```python
from build123d import *

# Parameters (mm, degrees)
SKETCH1_R           = 8.255
SKETCH1_R_2         = 5.715
BOSS_EXTRUDE1_DEPTH = 269.875
CUT_EXTRUDE1_DEPTH  = 271.127387865
SKETCH3_R           = 1.524
CUT_EXTRUDE2_DEPTH  = 271.127387865
SKETCH4_R           = 5.715
SKETCH4_R_2         = 5.08
BOSS_EXTRUDE2_DEPTH = 3.81


with BuildPart() as part:
    # Sketch1 → Boss-Extrude1 (new body)
    with BuildSketch(Plane(origin=(0, 0, 0), x_dir=(1, 0, 0), z_dir=(0, 1, 0))):
        with Locations(Location((0, 0, 0), (0, 0, 270))):
            Circle(SKETCH1_R)
        with Locations(Location((0, 0, 0), (0, 0, 270))):
            Circle(SKETCH1_R_2, mode=Mode.SUBTRACT)
    extrude(amount=BOSS_EXTRUDE1_DEPTH)

    # Sketch2 → Cut-Extrude1 (cut, through all)
    with BuildSketch(Plane(origin=(0, 0, 0), x_dir=(0, 0, -1), z_dir=(1, 0, 0))):
        Polygon((1.833087105, 260.35), (3.666174209, 263.525), (1.833087105, 266.7), (-1.833087105, 266.7), (-3.666174209, 263.525), (-1.833087105, 260.35), align=None)
    extrude(amount=-CUT_EXTRUDE1_DEPTH, mode=Mode.SUBTRACT)

    # Sketch3 → Cut-Extrude2 (cut, through all)
    with BuildSketch(Plane(origin=(0, 0, 0), x_dir=(0, 0, -1), z_dir=(1, 0, 0))):
        with Locations(Location((0, 263.525, 0), (0, 0, 180))):
            Circle(SKETCH3_R)
    extrude(amount=CUT_EXTRUDE2_DEPTH, mode=Mode.SUBTRACT)

    # Sketch4 → Boss-Extrude2 (add)
    with BuildSketch(Plane.XZ):
        with Locations(Location((0, 0, 0), (0, 0, 270))):
            Circle(SKETCH4_R)
        with Locations(Location((0, 0, 0), (0, 0, 270))):
            Circle(SKETCH4_R_2, mode=Mode.SUBTRACT)
    extrude(amount=-BOSS_EXTRUDE2_DEPTH)


solid = part.part
```
Geometry: final body of the model. Coordinates: model frame, mm. A direction names the side the tool comes from. Give positions to 0.01 mm unless a question says otherwise; leave off trailing zeros. Order: outer loops, then holes, each group sorted by start corner. A loop starts at its lowest first (then second) coordinate and runs counter-clockwise, first axis right, second up. Notation, with made-up numbers: (-18.5, 80.5) -> (40.5, 80.5) arc R27 ccw to (40.5, 107.5) -> close; hole circle Ø3 at (72, -29). An arc over 180 degrees is marked (long way). Write each question's results on one line, items separated by ' | '. Start each with the question number.
1) Section A-A (x = 0). Return loops of the section in (y, z) (3 decimals).
2) Set-up query: faces 4 (the flat face through (-2, 269.875, -6)), 5 (the cylindrical face through (5.666, 134.98, -0.744)). Return all of +Z, -Z, +X, -X, +Y, -Y with unobstructed straight access to the full face (end or side cutting, diameter ignored); none if empty.
3) Section B-B (y = 73). Return loops of the section in (x, z) (3 decimals), then the cut area to 3 significant figures.
4) Line query: line 1 (Y direction, x = 6.3, z = 0) (3 decimals); line 2 (Z direction, x = 6.5, y = 240); line 3 (X direction, y = 2.9, z = 0) (3 decimals). Output: solid intervals per line, ascending. Write a range as from..to.
5) Draft query along X for faces 1 (the cylindrical face through (5.037, 1.878, 0.661)), 2 (the cylindrical face through (-5.023, 133.048, -6.551)), 3 (the flat face through (-4, 0, 4)). Return one class per face: pulls with the +X half, pulls with the -X half, needs draft (parallel to the pull), parting line crosses it, or undercut.
6) First-contact query: pin 1 (5.5 mm diameter, centred on x = -0.5, z = 2.5, fed in from +Y); pin 2 (5 mm diameter, centred on y = 199, z = -6.5, fed in from +X); pin 3 (5 mm diameter, centred on x = 4, y = 169.5, fed in from +Z). Flat tips, straight axial feed; report the tip coordinate or a pass-through.
Calculated:
1) outline: (0, -8.255) -> (269.875, -8.255) -> (269.875, -5.715) -> (3.81, -5.715) -> (3.81, -5.08) -> (0, -5.08) -> close; (0, 5.08) -> (3.81, 5.08) -> (3.81, 5.715) -> (269.875, 5.715) -> (269.875, 8.255) -> (0, 8.255) -> close
2) face 4: +Z, -Z, +X, -X, +Y | face 5: +Y
3) outline: circle Ø16.51 at (0, 0); hole circle Ø11.43 at (0, 0) | area: 111 mm2
4) line 1: 0..262.001, 265.049..269.875 | line 2: -5.09..5.09 | line 3: -8.255..-5.08, 5.08..8.255
5) face 1: undercut | face 2: parting line crosses it | face 3: needs draft
6) pin 1: y = 3.81 | pin 2: x = 7.22 | pin 3: z = 8.12
